Build history of the part. All positions in model axes, mm. Give positions to 0.01 mm unless a question says otherwise; leave off trailing zeros. Loops run counter-clockwise (first coordinate to the right, second up) from the corner with the lowest first, then second, coordinate; pieces in that order, holes last. Notation, with made-up numbers: (67, -3.5) -> (74, -3.5) arc R24 ccw to (74, 13.5) -> close; hole circle Ø4 at (16, 57.25). An arc over 180 degrees is marked (long way). One line per question, with ' | ' between items. Start each with the question number.
(1) Drill centre lines: L1, parallel to X at y = -2.8, z = 0; L2, parallel to X at y = -0.1, z = 0; L3, parallel to X at y = 0.4, z = -2. Where is each one in solid material? Low to high. Write a range as from..to.
(2) Slice it at C-C, the plane z = -1. Write the cut outline in (x, y).
(3) Slice it at A-A, the plane y = 0. Write the cut outline in (x, z).
(4) Slice it at B-B, the plane x = -6. Write the cut outline in (y, z).
(5) Flat gauge pins, fed straight in: pin 1 Ø1 at (x, y) = (-3.5, 0.5) entering from -Z; pin 2 Ø2 at (x, z) = (-4.5, 1) entering from -Y. Where does each tip first touch, or does it go through?
(6) Mould opens along X. For faces 1 (the face through (19.477, -0.719, -0.15)), 2 (the face through (-10, 0, 0)), 3 (the face through (-4.93, -0.07, -1.5)) say: pulls with the +X half, pulls with the -X half, needs draft (parallel to the pull), parting line crosses it, or undercut.
(7) Slice it at D-D, the plane x = 3. Write the cut outline in (y, z).
Autodesk Inventor part; units mm, degrees
ref_plane "Start Plane" through (0, 0, 0) normal (1, 0, 0) x (0, 1, 0)
ref_plane "XZ Plane" through (0, 0, 0) normal (0, 1, 0) x (-1, 0, 0)
ref_plane "XY Plane" through (0, 0, 0) normal (0, 0, 1) x (1, 0, 0)
sketch "Sketch4" plane through (0, 0, 0) normal (1, 0, 0) x (0, 1, 0)
  circle A0 centre (0, 0) radius 3
  dimension "d11" = 6
extrude "Extrusion2" add sketch "Sketch4" along normal blind 22
sketch "Sketch5" plane through (22, 0, 0) normal (1, 0, 0) x (0, 0, -1)
  circle A0 centre (0, 0) radius 3
  line L0 (-2.5981, 1.5) -> (2.5981, 1.5)
  circle A1 centre (0, 0) radius 3
  dimension "d14" = 1.5
extrude "Extrusion3" cut sketch "Sketch5" against normal through all contours L0 A0 picked at (0.7274, 1.6862)
sketch "Sketch6" plane through (0, 0, 0) normal (-1, 0, 0) x (0, 0, 1)
  circle A0 centre (0, 0) radius 1.5
  dimension "d17" = 3
extrude "Extrusion4" add sketch "Sketch6" along normal blind 10
thread "Thread1"
sketch "Sketch7" plane through (22, 1.5, 2.5981) normal (0, 1, 0) x (1, 0, 0)
  circle A0 centre (-19, 2.5981) radius 0.5
  circle A1 centre (-3, 2.5981) radius 0.5
  point P0 (-22, 2.5981)
  dimension "d22" = 1
  dimension "d23" = 3
  dimension "d24" = 15
  dimension "d25" = 16
extrude "Extrusion5" cut sketch "Sketch7" against normal through all
equation "\"Length\" = 18"
properties part number "centre shaft" material "Steel, Mild"
Final values:
1) L1: 0..2.5, 3.5..18.5, 19.5..22 | L2: -10..2.5, 3.5..18.5, 19.5..22 | L3: 0..22
2) outline: (-10, -1.12) -> (0, -1.12) -> (0, -2.83) -> (22, -2.83) -> (22, 1.5) -> (0, 1.5) -> (0, 1.12) -> (-10, 1.12) -> close
3) outline: (-10, -1.5) -> (0, -1.5) -> (0, -3) -> (22, -3) -> (22, 3) -> (0, 3) -> (0, 1.5) -> (-10, 1.5) -> close; hole circle Ø1 at (3, 0); hole circle Ø1 at (19, 0)
4) outline: circle Ø3 at (0, 0)
5) pin 1: z = -1.5 | pin 2: y = -1.5
6) face 1: undercut | face 2: pulls with the -X half | face 3: needs draft
7) outline: (-2.96, -0.5) arc R3 ccw to (1.5, -2.6) -> (1.5, -0.5) -> close; (-2.96, 0.5) -> (1.5, 0.5) -> (1.5, 2.6) arc R3 ccw to start
